from build123d import *

# Parameters (mm, degrees)
F0_R     = 11.1633
F1_DEPTH = 58.42
F2_SIZE2 = 48.3329714275
F2_SIZE  = 5.08
F3_R     = 2.54


with BuildPart() as f1:
    # F0 (on Top) → F1 (new body)
    with BuildSketch(Plane.XY):
        Circle(F0_R)
    extrude(amount=F1_DEPTH)

    # F2
    f2_edges = [f1.edges().sort_by_distance(p)[0] for p in [
        (-11.1633, 0, 58.42),
    ]]
    f2_side = f1.faces().sort_by_distance((0, 0, 58.42))[0]
    chamfer(f2_edges, length=F2_SIZE, length2=F2_SIZE2, reference=f2_side)

    # F3
    f3_edges = [f1.edges().sort_by_distance(p)[0] for p in [
        (-6.0833, 0, 58.42),
    ]]
    fillet(f3_edges, radius=F3_R)


solid = f1.part
Build history of the part. All positions in model axes, mm. Round coordinates to 2 decimals unless told otherwise and drop trailing zeros. Write each loop counter-clockwise with the first axis right and the second up, starting at its lowest first coordinate (ties: lowest second). Pieces come first, ordered by that corner, then holes. Notation, with made-up numbers: (-11.5, 62) - (10.5, 62) arc R10 cw to (10.5, 78) - close; hole circle Ø9 at (73.5, 53). An arc over 180 degrees is marked (long way). One line per question, with ' | ' between items.
1. Band-saw the part on C-C, the plane z = 45.5. Write the cut outline in (x, y), and give its area (3 significant figures).
Results are:
outline: circle Ø14.88 at (0, 0) | area: 174 mm^2
2. Band-saw the part on A-A, the plane x = 0. Write the cut outline in (y, z), and give its area (3 significant figures).
Results are:
outline: (-11.16, 0) - (11.16, 0) - (11.16, 10.09) - (6.32, 56.15) arc R2.54 ccw to (3.8, 58.42) - (-3.8, 58.42) arc R2.54 ccw to (-6.32, 56.15) - (-11.16, 10.09) - close | area: 1,060 mm^2
3. Drop flat-ended pins along their axis: pin 1 Ø12 at (x, y) = (-6.5, 3) entering from -Z; pin 2 Ø2 at (x, z) = (-4.5, 34.5) entering from -Y; pin 3 Ø3 at (x, z) = (-5, 20) entering from +Y; pin 4 Ø4 at (y, z) = (-4.5, 36) entering from +X. Give the stop position or say it passes through.
Results are:
pin 1: z = 0 | pin 2: y = -7.87 | pin 3: y = 9.52 | pin 4: x = 8.1
4. Drill centre lines: line 1 along X through (y, z) = (3.5, 13); line 2 along Y through (x, z) = (0, 41); line 3 along X through (y, z) = (-0.25, 40.5). Where is each one in solid material? Low to high. Write a range as from..to.
Results are:
line 1: -10.28..10.28 | line 2: -7.91..7.91 | line 3: -7.96..7.96
5. Band-saw the part on D-D, the plane z = 32. Write the cut outline in (x, y).
Results are:
outline: circle Ø17.72 at (0, 0)
